Study the drawing (mm; zero at the part's minimum x, y, z) and answer. Coordinates: 2 decimals unless noted, no trailing zeros. Order: outer loops, then holes, each group sorted by start corner. A loop starts at its lowest first (then second) coordinate and runs counter-clockwise, first axis right, second up. Notation, with made-up numbers: M -19.75,24.5 L 18.25,24.5 A19 cw 18.25,52.5 Z; hole C 76,23.25 d1. An arc over 180 degrees is marked long. Use a Markdown table: item, result. Add a question column.
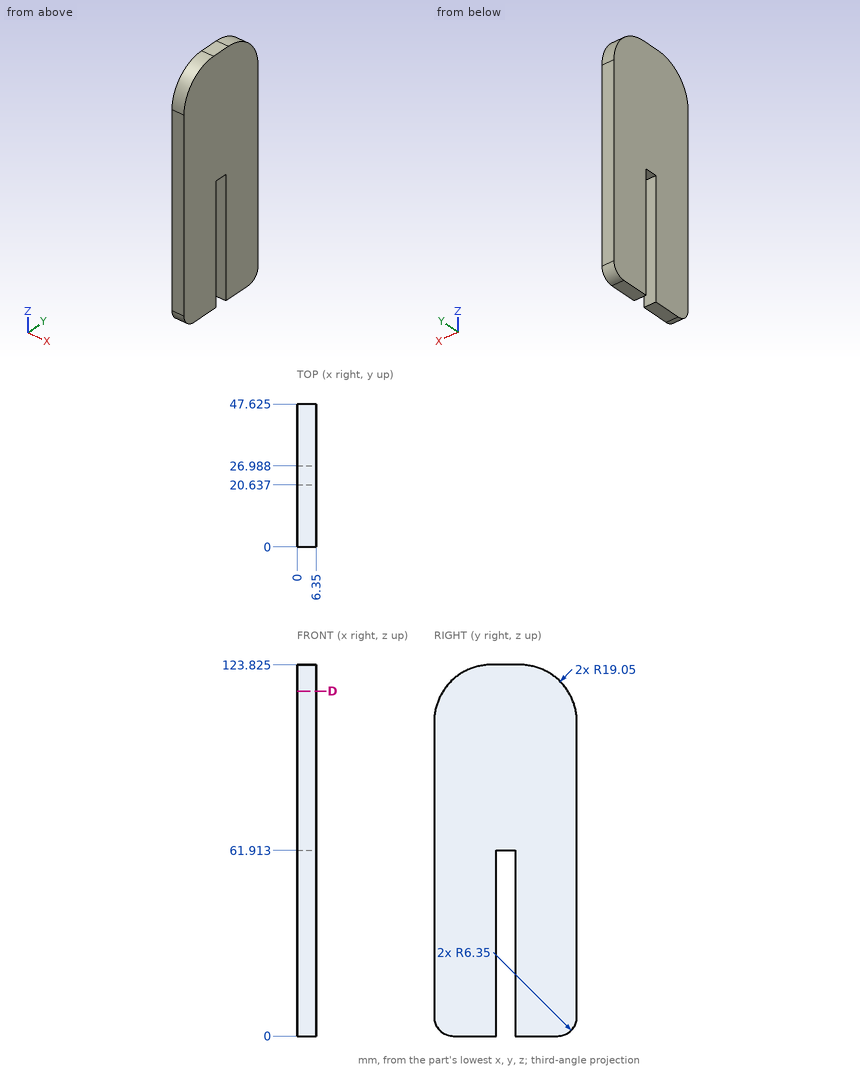
(1) A cutting plane is placed at D-D on z = 115. Write down the section's boundary in (x, y).
(2) Given P1, Ø3, axis at x = 3.5, y = 24.5, coming from the -Z side; P2, Ø1, axis at x = 2, y = 36, coming from the +Z side, each flat-ended and moving along its own axis, determine where each tip first touches the part or whether it passes through.
(3) Straight lines are drawn through the part: line 1 (Y direction, x = 4.5, z = 39) (1 decimal); line 2 (Z direction, x = 6.25, y = 29); line 3 (Z direction, x = 2.75, y = 32) (1 decimal). For each, find the intervals that lie inside material, in ascending order.
From the geometry:
| question | item | result |
|---|---|---|
| 1 | outline | M 0,2.98 L 6.35,2.98 L 6.35,44.65 L 0,44.65 Z |
| 2 | P1 | stops at z = 61.91 |
| 2 | P2 | stops at z = 122.52 |
| 3 | line 1 | y = 0 to 20.6, 27 to 47.6 |
| 3 | line 2 | z = 0 to 123.82 |
| 3 | line 3 | z = 0 to 123.5 |
